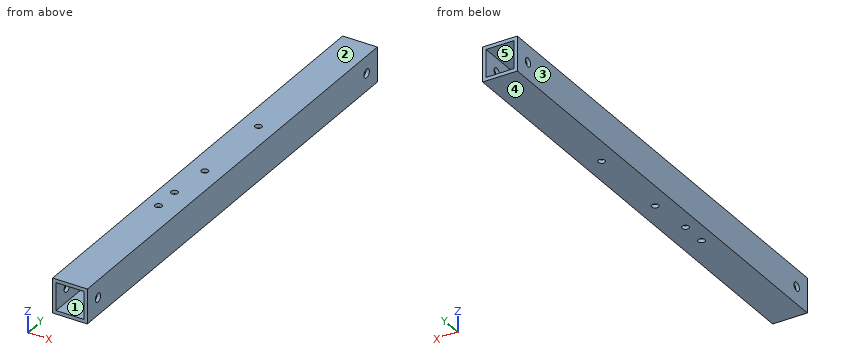
```python
from build123d import *

# Parameters (mm, degrees)
SKETCH1_W           = 25.4
SKETCH1_H           = 25.4
SKETCH1_W_2         = 20.32
SKETCH1_H_2         = 20.32
EXTRUDE_THIN1_DEPTH = 344.17
SKETCH2_R           = 2.4892
CUT_EXTRUDE1_DEPTH  = 26.4
SKETCH4_R           = 3.175
CUT_EXTRUDE3_DEPTH  = 26.4


with BuildPart() as part:
    # Sketch1 → Extrude-Thin1 (new body)
    with BuildSketch(Plane(origin=(0, 0, 0), x_dir=(1, 0, 0), z_dir=(0, 1, 0))):
        with Locations((12.7, 12.7)):
            Rectangle(SKETCH1_W, SKETCH1_H)
        with Locations((12.7, 12.7)):
            Rectangle(SKETCH1_W_2, SKETCH1_H_2, mode=Mode.SUBTRACT)
    extrude(amount=EXTRUDE_THIN1_DEPTH)

    # Sketch2 → Cut-Extrude1 (cut, through all)
    with BuildSketch(Plane(origin=(0, 0, -25.4), x_dir=(-1, 0, 0), z_dir=(0, 0, -1))):
        with Locations((-10.16, 109.1191)):
            Circle(SKETCH2_R)
        with Locations((-10.16, 128.1691)):
            Circle(SKETCH2_R)
        with Locations((-12.7, 160.02)):
            Circle(SKETCH2_R)
        with Locations((-12.7, 223.52)):
            Circle(SKETCH2_R)
    extrude(amount=-CUT_EXTRUDE1_DEPTH, mode=Mode.SUBTRACT)

    # Sketch4 → Cut-Extrude3 (cut, through all)
    with BuildSketch(Plane.ZY):
        with Locations((-12.7, 12.7)):
            Circle(SKETCH4_R)
        with Locations((-12.7, 331.47)):
            Circle(SKETCH4_R)
    extrude(amount=-CUT_EXTRUDE3_DEPTH, mode=Mode.SUBTRACT)


solid = part.part
```
Geometry: final body of the model. Coordinates: model frame, mm. Face numbers are marked on the shaded views. A direction names the side the tool comes from. Round coordinates to 2 decimals unless told otherwise and drop trailing zeros. Write each loop counter-clockwise with the first axis right and the second up, starting at its lowest first coordinate (ties: lowest second). Pieces come first, ordered by that corner, then holes.
Item 1: Mould query, pull axis Z, two halves, no side actions, for the marked faces 1, 2 and 3. Classes: +Z half, -Z half, draft (parallel to the pull), parting line (faces both ways), or undercut.
Item 2: Set-up query: the marked faces 4 and 5. Return all of +Z, -Z, +X, -X, +Y, -Y with unobstructed straight access to the full face (end or side cutting, diameter ignored); none if empty.
Item 3: Section query C-C (y = 12.7). Return loops of the section in (x, z) (3 decimals), plus the area to 3 significant figures.
Item 4: Material intervals for L1, parallel to Y at x = 10.16, z = -0.55; L2, parallel to Y at x = 12.7, z = -1.85; L3, parallel to X at y = 274.5, z = -10.25, sorted ascending.
Item 5: Section query A-A (z = -18.75). Return loops of the section in (x, y).
Item 6: Pin query (flat end, axial travel): P1, Ø4.5, axis at x = 12.7, y = 223.52, coming from the -Z side; P2, Ø7.5, axis at y = 331.47, z = -12.7, coming from the -X side. Return the tip coordinate at first contact, or that it passes through.
Item 7: Section query D-D (y = 51). Return loops of the section in (x, z).
Item 8: Section query B-B (x = 18). Return loops of the section in (y, z), plus the area to 3 significant figures.
Completed:
1. face 1: undercut
1. face 2: +Z half
1. face 3: draft
2. face 4: -Z, +X, -X, +Y, -Y
2. face 5: +Y, -Y
3. outline: (0, -25.4) - (25.4, -25.4) - (25.4, -15.875) - (22.86, -15.875) - (22.86, -22.86) - (2.54, -22.86) - (2.54, -15.875) - (0, -15.875) - close; (0, -9.525) - (2.54, -9.525) - (2.54, -2.54) - (22.86, -2.54) - (22.86, -9.525) - (25.4, -9.525) - (25.4, 0) - (0, 0) - close
3. area: 200 mm2
4. L1: y = 0 to 106.63, 111.61 to 125.68, 130.66 to 344.17
4. L2: y = 0 to 157.53, 162.51 to 221.03, 226.01 to 344.17
4. L3: x = 0 to 2.54, 22.86 to 25.4
5. outline: (0, 0) - (2.54, 0) - (2.54, 344.17) - (0, 344.17) - close; (22.86, 0) - (25.4, 0) - (25.4, 344.17) - (22.86, 344.17) - close
6. P1: passes through
6. P2: stops at x = 0
7. outline: (0, -25.4) - (25.4, -25.4) - (25.4, 0) - (0, 0) - close; hole (2.54, -22.86) - (22.86, -22.86) - (22.86, -2.54) - (2.54, -2.54) - close
8. outline: (0, -25.4) - (344.17, -25.4) - (344.17, -22.86) - (0, -22.86) - close; (0, -2.54) - (344.17, -2.54) - (344.17, 0) - (0, 0) - close
8. area: 1,750 mm2
